Could you check a few things on this model? Use its own coordinates, in mm. Give positions to 0.01 mm unless a question says otherwise; leave off trailing zeros. Order: outer loops, then holes, each group sorted by start corner. A loop starts at its lowest first (then second) coordinate and runs counter-clockwise, first axis right, second up. Notation, with made-up numbers: M 76.5,37 L 89.5,37 A22 ccw 89.5,64 Z; hole C 36.5,38 d9. An arc over 180 degrees is marked long. Use a Markdown table: item, result. Add a question column.
Item 1: Suppose I cut it at A-A on y = 0. Write out the boundary of the cut face in (x, z).
Item 2: Suppose I cut it at D-D on z = 102.5. Write out the boundary of the cut face in (x, y), plus the area to 3 significant figures.
Item 3: I'm going to push flat-ended pins straight in: pin 1 Ø1.3 at (y, z) = (20.5, 517.5) entering from +X; pin 2 Ø23 at (x, y) = (0, 0) entering from +Z; pin 3 Ø8 at (y, z) = (12.5, 76.5) entering from +X; pin 4 Ø4 at (x, z) = (-7.5, 421.5) entering from +Y. Where does each tip first touch, or does it pass through?
Item 4: Suppose I cut it at C-C on x = -10. Write out the boundary of the cut face in (y, z).
Item 5: Suppose I cut it at B-B on z = 480.5. Write out the boundary of the cut face in (x, y).
Item 6: If I drill on L1, parallel to Y at x = 0, z = 81; L2, parallel to X at y = 1.5, z = 157.5, over which ranges is the centre line in solid material (lowest first)? Write a range as from..to.
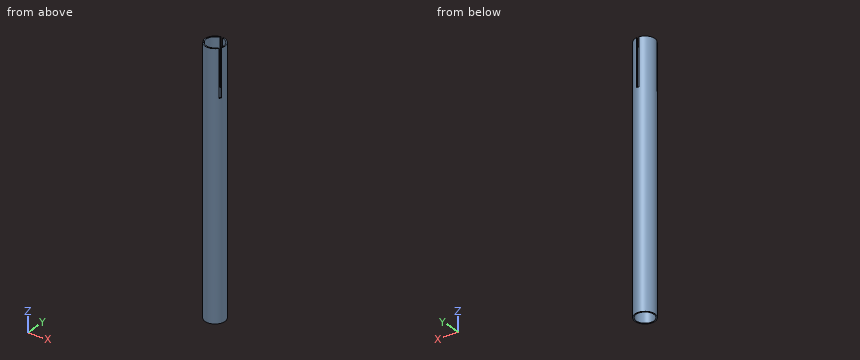
from build123d import *

# Parameters (mm, degrees)
SKETCH1_R               = 21.59
SKETCH1_R_2             = 19.05
BOSS_EXTRUDE1_DEPTH     = 558.8
CUT_EXTRUDE1_REACH      = 561.634
CUT_EXTRUDE1_END_RADIUS = 21.59
SKETCH2_W               = 5.08
SKETCH2_H               = 101.6
CIRPATTERN1_COUNT       = 3


with BuildPart() as part:
    # Sketch1 → Boss-Extrude1 (new body)
    with BuildSketch(Plane.XY):
        Circle(SKETCH1_R)
        Circle(SKETCH1_R_2, mode=Mode.SUBTRACT)
    extrude(amount=BOSS_EXTRUDE1_DEPTH)

    # Cut-Extrude1: up to this cylinder (the profile starts inside it)
    cut_extrude1_end = Plane(origin=(0, 0, 508), z_dir=(0, 0, -1)) * Cylinder(CUT_EXTRUDE1_END_RADIUS, 1167.448, mode=Mode.PRIVATE)
    # Sketch2 → Cut-Extrude1 (cut, up to the surface)
    with BuildSketch(Plane(origin=(0, 0, 0), x_dir=(1, 0, 0), z_dir=(0, 1, 0)), mode=Mode.PRIVATE) as cut_extrude1_sk1:
        with Locations((0, -508)):
            Rectangle(SKETCH2_W, SKETCH2_H)
    cut_extrude1_tool1 = extrude(cut_extrude1_sk1.sketch, amount=CUT_EXTRUDE1_REACH, mode=Mode.PRIVATE) & cut_extrude1_end
    cut_extrude1 = cut_extrude1_tool1.solids().sort_by_distance((0, 0, 508))[0]
    add(cut_extrude1, mode=Mode.SUBTRACT)

    # CirPattern1: Cut-Extrude1 ×3 about axis
    cirpattern1_axis = Axis((0, 0, 0), (0, 0, 1))
    for i in range(1, CIRPATTERN1_COUNT):
        add(cut_extrude1.rotate(cirpattern1_axis, i * 360 / CIRPATTERN1_COUNT), mode=Mode.SUBTRACT)


solid = part.part
Findings below:
| question | item | result |
|---|---|---|
| 1 | outline | M -21.59,0 L -19.05,0 L -19.05,558.8 L -21.59,558.8 Z; M 19.05,0 L 21.59,0 L 21.59,558.8 L 19.05,558.8 Z |
| 2 | outline | C 0,0 d43.18; hole C 0,0 d38.1 |
| 2 | area | 324 mm^2 |
| 3 | pin 1 | stops at x = 8.49 |
| 3 | pin 2 | passes through |
| 3 | pin 3 | stops at x = 19.85 |
| 3 | pin 4 | stops at y = 20.88 |
| 4 | outline | M -19.13,0 L -16.21,0 L -16.21,558.8 L -19.13,558.8 Z; M 16.21,0 L 19.13,0 L 19.13,558.8 L 16.21,558.8 Z |
| 5 | outline | M -19.84,-8.52 L -17.62,-7.24 A19.05 cw -2.54,18.88 L -2.54,21.44 A21.59 ccw Z; M -17.3,-12.92 A21.59 ccw 17.3,-12.92 L 15.08,-11.64 A19.05 cw -15.08,-11.64 Z; M 2.54,18.88 A19.05 cw 17.62,-7.24 L 19.84,-8.52 A21.59 ccw 2.54,21.44 Z |
| 6 | L1 | y = -21.59..-19.05, 19.05..21.59 |
| 6 | L2 | x = -21.54..-18.99, 18.99..21.54 |
